Verification items for this drawing (mm, ordinates from the low corner). Round coordinates to 2 decimals unless told otherwise and drop trailing zeros. Loops run counter-clockwise (first coordinate to the right, second up) from the corner with the lowest first, then second, coordinate; pieces in that order, holes last. Notation, with made-up numbers: M 25,-11.5 L 39,-11.5 A36 cw 39,23.5 Z; hole C 7.5,11 d3. An arc over 180 degrees is marked long. One line per item, written item: value.
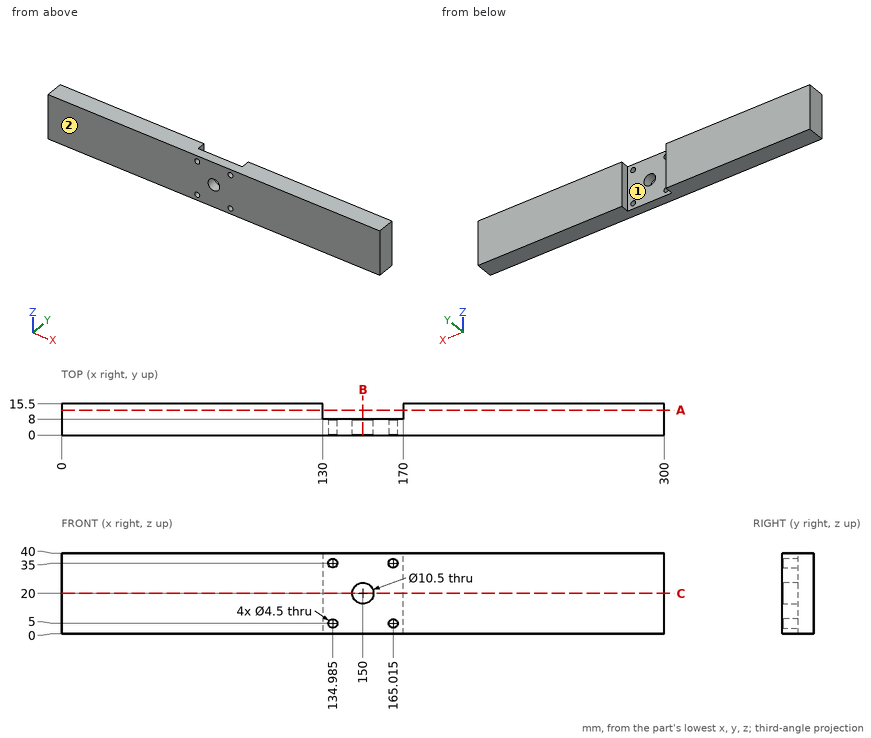
(1) Thickness scan on L1, parallel to X at y = 9.25, z = 12; L2, parallel to X at y = 4.25, z = 20; L3, parallel to Y at x = 133.5, z = 7.5. Record the ranges inside material, lowest first. Write a range as from..to.
Completed:
L1: x = 0..130, 170..300
L2: x = 0..144.75, 155.25..300
L3: y = 0..8
(2) Sectioned sample at A-A on y = 12.5. Enter the section's corners in (x, z), and give its area (3 significant figures).
Completed:
outline: M 0,0 L 130,0 L 130,40 L 0,40 Z; M 170,0 L 300,0 L 300,40 L 170,40 Z
area: 10,400 mm^2
(3) Sectioned sample at B-B on x = 150. Enter the section's corners in (y, z).
Completed:
outline: M 0,0 L 8,0 L 8,14.75 L 0,14.75 Z; M 0,25.25 L 8,25.25 L 8,40 L 0,40 Z
(4) Mould release check, pull along X, two halves, no side actions. Record for the marked faces 1 and 2: +X half, -X half, draft (parallel to the pull), parting line (faces both ways), or undercut.
Completed:
face 1: undercut
face 2: draft
(5) Sectioned sample at C-C on z = 20. Enter the section's corners in (x, y), and give its area (3 significant figures).
Completed:
outline: M 0,0 L 144.75,0 L 144.75,8 L 130,8 L 130,15.5 L 0,15.5 Z; M 155.25,0 L 300,0 L 300,15.5 L 170,15.5 L 170,8 L 155.25,8 Z
area: 4,270 mm^2
(6) Depth check by flat-ended pin: pin 1 Ø2.5 at (x, z) = (134.985, 5) entering from +Y; pin 2 Ø3 at (x, y) = (122.5, 8) entering from -Z. Enter the tip coordinate at first touch or a pass-through.
Completed:
pin 1: passes through
pin 2: stops at z = 0
